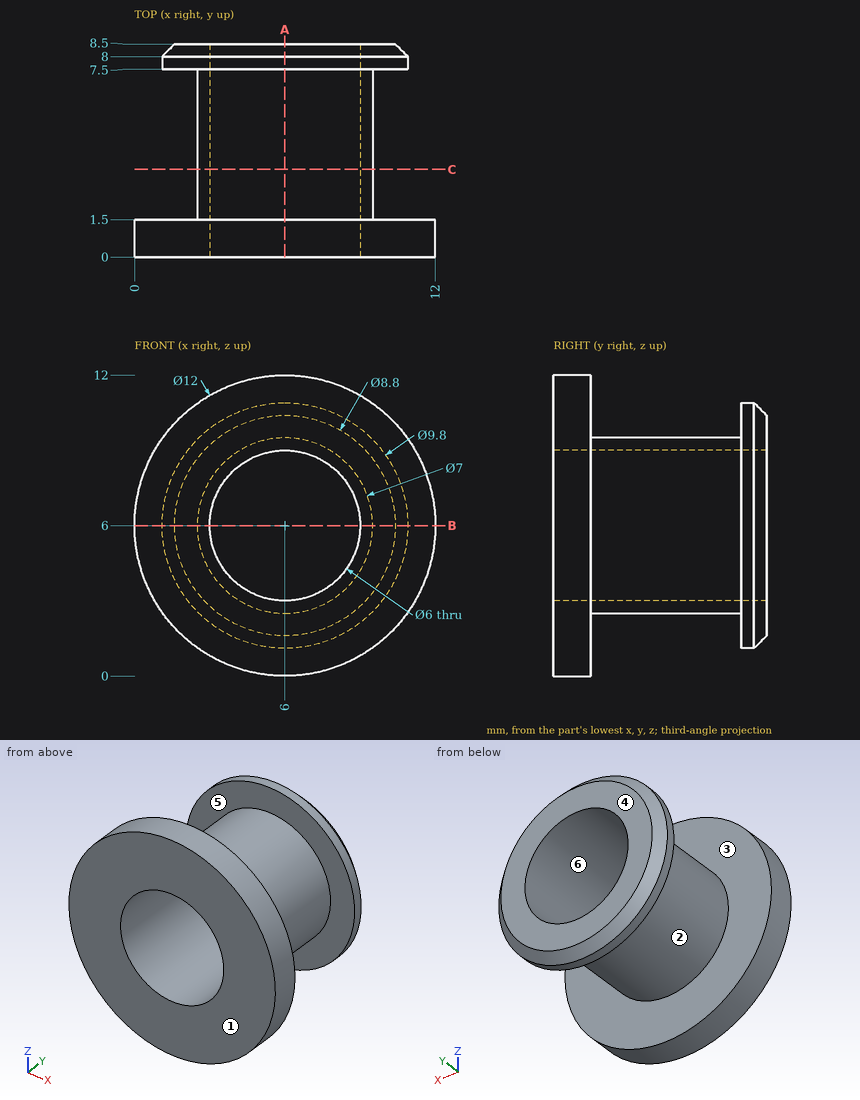
Design review of the part shown in the three views and the two pictorial views. Dimensions are in mm from the part's minimum x, y and z. A direction names the side the tool comes from. Round coordinates to 2 decimals unless told otherwise and drop trailing zeros. Loops run counter-clockwise (first coordinate to the right, second up) from the corner with the lowest first, then second, coordinate; pieces in that order, holes last.
Q1. Machinability: for the marked faces 1 and 2, which of the approach directions +Z, -Z, +X, -X, +Y, -Y give a long, thin tool a straight path to every point of the face, cutting with its end or side? Answer none if there is none.
Result sheet:
face 1: +Z, -Z, +X, -X, -Y
face 2: none
Q2. To check wall thickness, follow line 1 along X through (y, z) = (3.25, 6); line 2 along Y through (x, z) = (2.75, 7.5); line 3 along Y through (x, z) = (10.5, 8.25). State the ranges of each line that lie inside material, in increasing order.
Result sheet:
line 1: x = 2.5 to 3, 9 to 9.5
line 2: y = 0 to 1.5, 7.5 to 8.5
line 3: y = 0 to 1.5
Q3. Mouldability with a two-part tool opening along Y and no side actions: class the marked faces 3, 4, 5 and 6 as +Y half, -Y half, draft (parallel to the pull), parting line (faces both ways), or undercut.
Result sheet:
face 3: undercut
face 4: +Y half
face 5: undercut
face 6: draft
Q4. Insertion check: pin 1 Ø5.5 at (x, z) = (6, 6) entering from -Y; pin 2 Ø1.5 at (y, z) = (6.5, 2.5) entering from -X. Each pin has a flat end and moves straight along its axis. Give the tip position at first contact, or say it passes through.
Result sheet:
pin 1: passes through
pin 2: stops at x = 3.83
Q5. Add section B-B on z = 6. Write out the cut boundary in (x, y).
Result sheet:
outline: (0, 0) - (3, 0) - (3, 8.5) - (1.6, 8.5) - (1.1, 8) - (1.1, 7.5) - (2.5, 7.5) - (2.5, 1.5) - (0, 1.5) - close; (9, 0) - (12, 0) - (12, 1.5) - (9.5, 1.5) - (9.5, 7.5) - (10.9, 7.5) - (10.9, 8) - (10.4, 8.5) - (9, 8.5) - close
Q6. Add section C-C on y = 3.5. Write out the cut boundary in (x, z), plus the area to 3 significant figures.
Result sheet:
outline: circle Ø7 at (6, 6); hole circle Ø6 at (6, 6)
area: 10.2 mm2
Q7. Add section A-A on x = 6. Write out the cut boundary in (y, z).
Result sheet:
outline: (0, 0) - (1.5, 0) - (1.5, 2.5) - (7.5, 2.5) - (7.5, 1.1) - (8, 1.1) - (8.5, 1.6) - (8.5, 3) - (0, 3) - close; (0, 9) - (8.5, 9) - (8.5, 10.4) - (8, 10.9) - (7.5, 10.9) - (7.5, 9.5) - (1.5, 9.5) - (1.5, 12) - (0, 12) - close
